Geometry check sheet. Reference: the model listing, model coordinates, mm. A direction names the side the tool comes from. Give positions to 0.01 mm unless a question says otherwise; leave off trailing zeros. Loops run counter-clockwise (first coordinate to the right, second up) from the corner with the lowest first, then second, coordinate; pieces in that order, holes last. Notation, with made-up numbers: (7, 54) -> (46, 54) arc R17 cw to (46, 84) -> close; hole circle Ø11 at (-14, -6). An arc over 180 degrees is marked (long way). Write each question's results on one line, items separated by ' | '. Start each with the question number.
1) Sectioned sample at C-C on x = 3.5. Count the separate pieces of the cut face and the enclosed holes in it, then the cut area to 3 significant figures.
2) Sectioned sample at A-A on z = 84.5. Record the cut outline in (x, y), then the cut area to 3 significant figures.
3) Draft check along Z on faces 6 (the face through (-4.626, -8.061, 91.044)), 7 (the face through (-1, 65.221, -97)). Enter one of: pulls with the +Z half, pulls with the -Z half, needs draft (parallel to the pull), parting line crosses it, or undercut.
4) Set-up check for faces 1 (the face through (-29.382, 61.418, -94.907)), 2 (the face through (28.91, 61.42, -94.76)), 3 (the face through (-33.891, 29.724, 82.544)), 4 (the face through (-81.837, 27.195, 43.361)), 5 (the face through (-1, 65.221, 98)): record each of +Z, -Z, +X, -X, +Y, -Y from which the full face is reachable in a straight line by a thin tool's end or side.
5) Sectioned sample at D-D on z = -81. Record the cut outline in (x, y).
6) Scan lines: line 1 (X direction, y = 49, z = -1); line 2 (Y direction, x = -40.5, z = -18); line 3 (Z direction, x = -44.5, y = -5.5). Record each from-to range of solid material in increasing order. Write a range as from..to.
7) Depth check by flat-ended pin: pin 1 (2 mm diameter, centred on y = 55.5, z = -5.5, fed in from -X); pin 2 (10 mm diameter, centred on y = 56, z = 16, fed in from -X); pin 3 (4 mm diameter, centred on y = 56.5, z = 82.5, fed in from +X). Enter the tip coordinate at first touch or a pass-through.
```python
from build123d import *

# Parameters (mm, degrees)
SKETCH2_R           = 61.5
BOSS_EXTRUDE1_DEPTH = 50
SKETCH6_R           = 59
CUT_EXTRUDE1_DEPTH  = 48
SKETCH7_R           = 6
CUT_EXTRUDE4_DEPTH  = 2
SKETCH9_R           = 21
CUT_EXTRUDE5_DEPTH  = 3
BOSS_EXTRUDE2_START = -5
BOSS_EXTRUDE2_DEPTH = 5.0001
SCALE2_SCALE        = 1.5


# Read off the part's stored shape, not the designer's step: Boss-Extrude2
with BuildPart() as part:
    # Sketch2 → Boss-Extrude1 (new body)
    with BuildSketch(Plane(origin=(0, 0, 0), x_dir=(1, 0, 0), z_dir=(0, 1, 0))):
        with Locations(Location((0, 0, 0), (0, 0, 270))):
            Circle(SKETCH2_R)
    extrude(amount=BOSS_EXTRUDE1_DEPTH)

    # Sketch6 → Cut-Extrude1 (cut)
    with BuildSketch(Plane(origin=(0, 50, 0), x_dir=(1, 0, 0), z_dir=(0, 1, 0))):
        with Locations(Location((0, 0, 0), (0, 0, 270))):
            Circle(SKETCH6_R)
    extrude(amount=-CUT_EXTRUDE1_DEPTH, mode=Mode.SUBTRACT)

    # Sketch7 → Cut-Extrude4 (cut)
    with BuildSketch(Plane(origin=(0, 0, 0), x_dir=(1, 0, 0), z_dir=(0, 1, 0))):
        with Locations(Location((0, 0, 0), (0, 0, 270))):
            Circle(SKETCH7_R)
    extrude(amount=CUT_EXTRUDE4_DEPTH, mode=Mode.SUBTRACT)

    # Sketch9 → Cut-Extrude5 (cut)
    with BuildSketch(Plane(origin=(0, 0, 0), x_dir=(1, 0, 0), z_dir=(0, 1, 0))):
        with Locations(Location((0, -39.395608547, 0), (0, 0, 244.065435775))):
            Circle(SKETCH9_R)
    extrude(amount=CUT_EXTRUDE5_DEPTH, mode=Mode.SUBTRACT)

    # Boss-Extrude2 outline → Boss-Extrude2 (add)
    with BuildSketch(Plane(origin=(0, 50, 0), x_dir=(1, 0, 0), z_dir=(0, 1, 0)).offset(BOSS_EXTRUDE2_START)):
        with BuildLine():
            ThreePointArc((18.731112888, -58.578113745), (-0.20418242, -61.499661052), (-19.119661096, -58.452446994))
            Line((-19.119661096, -58.452446994), (-20.049464932, -68.999980107))
            Line((-20.049464932, -68.999980107), (19.825959412, -68.968020016))
            Line((19.825959412, -68.968020016), (18.731112888, -58.578113745))
        make_face()
        with BuildLine():
            Line((-20.049464932, 68.999980107), (-19.119661096, 58.452446994))
            ThreePointArc((-19.119661096, 58.452446994), (-0.20418242, 61.499661052), (18.731112888, 58.578113745))
            Line((18.731112888, 58.578113745), (19.825959412, 68.968020016))
            Line((19.825959412, 68.968020016), (-20.049464932, 68.999980107))
        make_face()
    extrude(amount=BOSS_EXTRUDE2_DEPTH)


with BuildPart() as part_1:
    # Scale2: scaled about (-0.009677872, 19.559028085, -1.585736767)
    add(part.part.scale(SCALE2_SCALE).moved(Location((0.004838936, -9.779514043, 0.792868383))))


solid = part_1.part
```
Result:
1) separate pieces: 3 | enclosed holes: 0 | area: 1,020 mm^2
2) outline: (-38.77, -9.78) -> (-19.65, -9.78) -> (-19.65, -6.78) -> (-28.72, -6.78) -> (-28.72, 65.22) -> (-38.77, 65.22) -> close; (19.66, -9.78) -> (38.78, -9.78) -> (38.78, 65.22) -> (28.73, 65.22) -> (28.73, -6.78) -> (19.66, -6.78) -> close | area: 1,560 mm^2
3) face 6: undercut | face 7: needs draft
4) face 1: -X, +Y, -Y | face 2: +X, +Y, -Y | face 3: +Y | face 4: -Y | face 5: +Z, -Z, +X, -X, +Y
5) outline: (-42.66, -9.78) -> (42.67, -9.78) -> (42.67, 65.22) -> (33.8, 65.22) -> (33.8, -6.78) -> (-33.79, -6.78) -> (-33.79, 65.22) -> (-42.66, 65.22) -> close
6) line 1: -92.23..-88.48, 88.49..92.24 | line 2: -9.78..-6.78 | line 3: -80.01..-75.7, 77.29..81.6
7) pin 1: x = -92.09 | pin 2: x = -91.68 | pin 3: x = 46.45
